Design review of the part built by this model. Coordinates are the model's own, in mm. Coordinates: 2 decimals unless noted, no trailing zeros. Write each loop counter-clockwise with the first axis right and the second up, starting at its lowest first coordinate (ties: lowest second). Pieces come first, ordered by that corner, then holes. Notation, with made-up numbers: (64, 66.5) -> (107, 66.5) arc R17 cw to (107, 77.5) -> close; hole circle Ø7 at (-39.75, 85). An arc over 180 degrees is marked (long way). Answer in a Markdown table with one row per item. Add a question column.
Item 1: To check wall thickness, follow line 1 (X direction, y = -4.75, z = 1340); line 2 (X direction, y = 5, z = 560); line 3 (Y direction, x = 8.5, z = 231). State the ranges of each line that lie inside material, in increasing order.
Item 2: Take a section at A-A, the plane z = 830. Write out the cut boundary in (x, y), and give its area (3 significant figures).
Item 3: Take a section at B-B, the plane x = 0. Give the number of separate pieces and of enclosed holes in the cut face, and give its area (3 significant figures).
Item 4: Clearance check with a flat-ended pin moving along its axis: P1, Ø5, axis at x = 1, z = 200, coming from the +Y side. State where the tip first meets the part, or that it passes through.
Autodesk Fusion 360 part; units mm, degrees
sketch "Sketch1" plane through (0, 0, 0) normal (0, 0, 1) x (1, 0, 0)
  line L0 (10, -8.75) -> (-10, -8.75)
  line L1 (10, -8.75) -> (10, -4.15)
  line L2 (0, 0) -> (12.5, 0) construction
  line L3 (10, -4.15) -> (5.85, 0)
  line L4 (5.85, 0) -> (5.85, 2)
  line L5 (9.9, -8.75) -> (10, -8.65)
  line L6 (9.9, -8.75) -> (10.0414, -8.75) construction
  line L7 (10, 6.45) -> (10, 4.95)
  line L8 (10, 6.45) -> (6.5, 8.75)
  line L9 (10, 4.95) -> (5.85, 2)
  line L10 (-10, -8.75) -> (10, -8.75) construction
  line L11 (-9.9, -8.75) -> (-10, -8.65)
  line L12 (-10, -8.75) -> (-10, -4.15)
  line L13 (-10, -4.15) -> (-5.85, 0)
  line L14 (-5.85, 0) -> (-5.85, 2)
  line L15 (-10, 4.95) -> (-5.85, 2)
  line L16 (-10, 6.45) -> (-6.5, 8.75)
  line L17 (-10, 6.45) -> (-10, 4.95)
  line L18 (-6.5, 8.75) -> (6.5, 8.75)
  dimension "d8" = 20
  dimension "d9" = 4.6
  dimension "d16" = 45
  dimension "d18" = 1.5
  dimension "d19" = 2
  dimension "d20" = 2
  dimension "d21" = 1.5
  dimension "d22" = 4.6
  dimension "d23" = 13
extrude "Extrude1" add sketch "Sketch1" along normal blind 1500 contours L0 L1 L3 L4 L5 L7 L8 L9 L11 L12 L13 L14 L15 L16 L17 L18
sketch "Sketch2" plane through (0, 8.75, 0) normal (0, 1, 0) x (-1, 0, 0)
  line L0 (-6.5, 0) -> (6.5, 0)
  line L1 (6.5, 0) -> (6.5, 1500)
  line L2 (6.5, 1500) -> (-6.5, 1500)
  line L3 (-6.5, 1500) -> (-6.5, 0)
  line L4 (0, 0) -> (0, 20) construction
  circle A0 centre (0, 20) radius 4.75
  circle A1 centre (0, 20) radius 3
  dimension "d26" = 20
  dimension "d27" = 9.5
  dimension "d28" = 6
extrude "Extrude2" cut sketch "Sketch2" against normal blind 8.5 contours A0 | A1
extrude "Extrude3" cut sketch "Sketch2" against normal blind 17.5 contours A1
pattern_linear "R-Pattern1" count 25 spacing 60 along (0, 0, 1) of "Extrude3", "Extrude2"
Answers:
| question | item | result |
|---|---|---|
| 1 | line 1 | x = -10 to -3, 3 to 10 |
| 1 | line 2 | x = -10 to -4.75, 4.75 to 10 |
| 1 | line 3 | y = -8.75 to -2.65, 3.88 to 7.44 |
| 2 | outline | (-10, -8.65) -> (-9.9, -8.75) -> (9.9, -8.75) -> (10, -8.65) -> (10, -4.15) -> (5.85, 0) -> (5.85, 2) -> (10, 4.95) -> (10, 6.45) -> (6.5, 8.75) -> (-6.5, 8.75) -> (-10, 6.45) -> (-10, 4.95) -> (-5.85, 2) -> (-5.85, 0) -> (-10, -4.15) -> close |
| 2 | area | 296 mm^2 |
| 3 | separate pieces | 26 |
| 3 | enclosed holes | 0 |
| 3 | area | 22,900 mm^2 |
| 4 | P1 | stops at y = 0.25 |
